```python
from build123d import *

# Parameters (mm, degrees)
BOSS_EXTRUDE1_DEPTH = 20
SKETCH3_W           = 10
SKETCH3_H           = 35
CUT_EXTRUDE1_DEPTH  = 48.5
SKETCH4_R           = 10
CUT_EXTRUDE2_DEPTH  = 21


with BuildPart() as part:
    # Sketch1 → Boss-Extrude1 (new body)
    with BuildSketch(Plane.XY):
        with BuildLine():
            Line((-5, -22.5), (5, -22.5))
            Line((5, -22.5), (5, 22.5))
            Line((5, 22.5), (10, 22.5))
            ThreePointArc((10, 22.5), (15.132819854, 38.37888203), (29.113715132, 47.490374848))
            ThreePointArc((29.113715132, 47.490374848), (41.674629404, 69.811001246), (18.518518519, 80.755472857))
            ThreePointArc((18.518518519, 80.755472857), (0, 77.19968102), (-18.518518519, 80.755472857))
            ThreePointArc((-18.518518519, 80.755472857), (-41.674629404, 69.811001246), (-29.113715132, 47.490374848))
            ThreePointArc((-29.113715132, 47.490374848), (-15.132819854, 38.37888203), (-10, 22.5))
            Line((-10, 22.5), (-5, 22.5))
            Line((-5, 22.5), (-5, -22.5))
        make_face()
    extrude(amount=BOSS_EXTRUDE1_DEPTH)

    # Sketch3 → Cut-Extrude1 (cut, through all)
    with BuildSketch(Plane(origin=(5, 0, 0), x_dir=(0, 0, -1), z_dir=(1, 0, 0))):
        with Locations((-10, -5)):
            Rectangle(SKETCH3_W, SKETCH3_H)
    extrude(amount=-CUT_EXTRUDE1_DEPTH, mode=Mode.SUBTRACT)

    # Sketch4 → Cut-Extrude2 (cut, through all)
    with BuildSketch(Plane(origin=(0, 0, 0), x_dir=(-1, 0, 0), z_dir=(0, 0, -1))):
        with Locations((-25, 64.5)):
            Circle(SKETCH4_R)
        with Locations((25, 64.5)):
            Circle(SKETCH4_R)
    extrude(amount=-CUT_EXTRUDE2_DEPTH, mode=Mode.SUBTRACT)


solid = part.part
```
Part model, mm, in its own coordinate system. A direction names the side the tool comes from. Round coordinates to 2 decimals unless told otherwise and drop trailing zeros. Order: outer loops, then holes, each group sorted by start corner. A loop starts at its lowest first (then second) coordinate and runs counter-clockwise, first axis right, second up. Notation, with made-up numbers: M 23.25,-27.75 L 32.25,-27.75 A27 ccw 32.25,6.25 Z; hole C 3.25,24.5 d9. An arc over 180 degrees is marked long. Answer in a Markdown table with one row per item. Add a question column.
Q1. Wall check: L1, parallel to Z at x = 4, y = -12.5; L2, parallel to X at y = 71.5, z = 5.25; L3, parallel to Y at x = -25, z = 13.5. Give the ranges that are in metal, low to high. Write a range as from..to.
Q2. Mould opens along X. For faces 1 (the face through (15.763, 60.67, 9.86)), 2 (the face through (-1, 54, 20)), 3 (the face through (5, 5, 3)) say: +X half, -X half, draft (parallel to the pull), parting line (faces both ways), or undercut.
Q3. Cut at A-A on y = -12. Give the cut face in (x, z), and give its area (3 significant figures).
Q4. Cut at C-C on x = 22. Give the cut face in (y, z), and give its area (3 significant figures).
Q5. Cut at D-D on y = 64.5. Give the cut face in (x, z), and give its area (3 significant figures).
Q6. Cut at B-B on z = 13.5. Give the cut face in (x, y).
Q7. Pin check, flat tips, straight feed: pin 1 (1 mm diameter, centred on x = 0.5, z = 7, fed in from -Y); pin 2 (12 mm diameter, centred on x = 25, y = 64.5, fed in from -Z); pin 3 (12 mm diameter, centred on y = 46, z = 6, fed in from -X); pin 4 (10 mm diameter, centred on x = 1, z = 2.5, fed in from +Y). Stop position of each tip, or through.
Q8. 3-axis set-ups, long thin cutter, end or side, ignore diameter. For faces 4 (the face through (0, -5, 5)), 5 (the face through (0.3, 77.2, 9.9)), 6 (the face through (-5, 5, 3)), 7 (the face through (7, 22.5, 10)): which of +Z, -Z, +X, -X, +Y, -Y reach the whole face in a straight line?
Established:
| question | item | result |
|---|---|---|
| 1 | L1 | z = 0..5, 15..20 |
| 1 | L2 | x = -41.04..-32.14, -17.86..17.86, 32.14..41.04 |
| 1 | L3 | y = 46.11..54.5, 74.5..82 |
| 2 | face 1 | undercut |
| 2 | face 2 | draft |
| 2 | face 3 | +X half |
| 3 | outline | M -5,0 L 5,0 L 5,5 L -5,5 Z; M -5,15 L 5,15 L 5,20 L -5,20 Z |
| 3 | area | 100 mm2 |
| 4 | outline | M 44.55,0 L 54.96,0 L 54.96,20 L 44.55,20 Z; M 74.04,0 L 81.74,0 L 81.74,20 L 74.04,20 Z |
| 4 | area | 362 mm2 |
| 5 | outline | M -42.5,0 L -35,0 L -35,20 L -42.5,20 Z; M -15,0 L 15,0 L 15,20 L -15,20 Z; M 35,0 L 42.5,0 L 42.5,20 L 35,20 Z |
| 5 | area | 900 mm2 |
| 6 | outline | M -29.11,47.49 A25 cw -10,22.5 L -5,22.5 L -5,12.5 L 5,12.5 L 5,22.5 L 10,22.5 A25 cw 29.11,47.49 A17.5 ccw long 18.52,80.76 A50 cw -18.52,80.76 A17.5 ccw long Z; hole C -25,64.5 d20; hole C 25,64.5 d20 |
| 7 | pin 1 | stops at y = 12.5 |
| 7 | pin 2 | passes through |
| 7 | pin 3 | stops at x = -37.25 |
| 7 | pin 4 | stops at y = 77.56 |
| 8 | face 4 | +X, -X, -Y |
| 8 | face 5 | +Z, -Z, +Y |
| 8 | face 6 | +Z, -Z, -X, -Y |
| 8 | face 7 | +Z, -Z, +X, -Y |
